Part model, mm, in its own coordinate system. A direction names the side the tool comes from. Give positions to 0.01 mm unless a question says otherwise; leave off trailing zeros. Write each loop counter-clockwise with the first axis right and the second up, starting at its lowest first coordinate (ties: lowest second). Pieces come first, ordered by that corner, then holes. Notation, with made-up numbers: M 82,75.25 L 111,75.25 A19 ccw 111,98.25 Z; hole C 35.5,22.5 d6. An arc over 180 degrees is marked long. Use CSV: the item, a comma, the result in double quotes. Start each with the question number.
Item 1: Cut at D-D (x = -14). List the corners of the cut face in (y, z), then the cut area to 3 significant figures.
Item 2: Cut at C-C (z = -1). List the corners of the cut face in (x, y).
Item 3: Mould opens along X. For faces 4 (the flat face through (19.646, 13.282, 3.535)), 5 (the flat face through (13.328, 19.691, 3.535)), 6 (the flat face through (19, -19, 1)), 7 (the cylindrical face through (-0.59, 4.46, -5.49)) say: released by +X, released by -X, zero draft, split by the parting line, or undercut.
Item 4: Pin check, flat tips, straight feed: pin 1 (18 mm diameter, centred on x = -3, y = -3, fed in from +Z); pin 2 (11 mm diameter, centred on x = 16.5, y = -19, fed in from -Z); pin 3 (1.5 mm diameter, centred on y = 16, z = 2.5, fed in from +X); pin 4 (3 mm diameter, centred on x = 17.75, y = 17.75, fed in from -Z). Stop position of each tip, or through.
Item 5: Drill centre lines: line 1 (X direction, y = -19.5, z = 2.5); line 2 (Y direction, x = 0, z = -1.4); line 3 (Z direction, x = -12.5, y = 2). Where is each one in solid material? Low to high. Write a range as [from, to].
Item 6: Which spindle directions (+Z, -Z, +X, -X, +Y, -Y) get a long thin tool onto all of the face, cutting with end or side? Do faces 1 (the cylindrical face through (-2.343, 17.847, 3.535)), 2 (the conical face through (21.2, -0.2, 5.8)), 3 (the flat face through (-19.5, 18.4, 1)). Say none if no direction does.
Item 7: Cut at A-A (y = 0). List the corners of the cut face in (x, z), then the cut area to 3 significant figures.
from build123d import *

# Parameters (mm, degrees)
SKETCH1_R           = 22
BOSS_EXTRUDE1_DEPTH = 6
CHAMFER1_SIZE       = 1
SKETCH8_R           = 1.6
BOSS_EXTRUDE2_DEPTH = 5
SKETCH9_R           = 18
CUT_EXTRUDE1_DEPTH  = 5
SKETCH10_R          = 8.5
CUT_EXTRUDE2_DEPTH  = 6
SKETCH11_R          = 4.5
CUT_EXTRUDE3_DEPTH  = 1


with BuildPart() as part:
    # Sketch1 → Boss-Extrude1 (new, symmetric)
    with BuildSketch(Plane.XY):
        Circle(SKETCH1_R)
    extrude(amount=BOSS_EXTRUDE1_DEPTH, both=True)

    # Chamfer1
    chamfer1_edges = [part.edges().sort_by_distance(p)[0] for p in [
        (-22, 0, 6),
    ]]
    chamfer(chamfer1_edges, length=CHAMFER1_SIZE)

    # Sketch8 → Boss-Extrude2 (add)
    # profile 1 of 4: a face of its own
    with BuildSketch(Plane.XY.offset(6)):
        with BuildLine():
            Line((20.930360723, -14.566399692), (17.68629022, -11.322329189))
            Line((17.68629022, -11.322329189), (11.322329189, -17.68629022))
            Line((11.322329189, -17.68629022), (14.566399692, -20.930360723))
            ThreePointArc((14.566399692, -20.930360723), (20.930360723, -20.930360723), (20.930360723, -14.566399692))
        make_face()
        with Locations((17.748380208, -17.748380208)):
            Circle(SKETCH8_R, mode=Mode.SUBTRACT)
    # profile 2 of 4: a face of its own
    with BuildSketch(Plane.XY.offset(6)):
        with BuildLine():
            Line((14.566399692, 20.930360723), (11.322329189, 17.68629022))
            Line((11.322329189, 17.68629022), (17.68629022, 11.322329189))
            Line((17.68629022, 11.322329189), (20.930360723, 14.566399692))
            ThreePointArc((20.930360723, 14.566399692), (20.930360723, 20.930360723), (14.566399692, 20.930360723))
        make_face()
        with Locations((17.748380208, 17.748380208)):
            Circle(SKETCH8_R, mode=Mode.SUBTRACT)
    # profile 3 of 4: a face of its own
    with BuildSketch(Plane.XY.offset(6)):
        with BuildLine():
            Line((-14.566399692, -20.930360723), (-11.322329189, -17.68629022))
            Line((-11.322329189, -17.68629022), (-17.68629022, -11.322329189))
            Line((-17.68629022, -11.322329189), (-20.930360723, -14.566399692))
            ThreePointArc((-20.930360723, -14.566399692), (-20.930360723, -20.930360723), (-14.566399692, -20.930360723))
        make_face()
        with Locations((-17.748380208, -17.748380208)):
            Circle(SKETCH8_R, mode=Mode.SUBTRACT)
    # profile 4 of 4: a face of its own
    with BuildSketch(Plane.XY.offset(6)):
        with BuildLine():
            Line((-20.930360723, 14.566399692), (-17.68629022, 11.322329189))
            Line((-17.68629022, 11.322329189), (-11.322329189, 17.68629022))
            Line((-11.322329189, 17.68629022), (-14.566399692, 20.930360723))
            ThreePointArc((-14.566399692, 20.930360723), (-20.930360723, 20.930360723), (-20.930360723, 14.566399692))
        make_face()
        with Locations((-17.748380208, 17.748380208)):
            Circle(SKETCH8_R, mode=Mode.SUBTRACT)
    extrude(amount=-BOSS_EXTRUDE2_DEPTH)

    # Sketch9 → Cut-Extrude1 (cut)
    with BuildSketch(Plane.XY.offset(6)):
        Circle(SKETCH9_R)
    extrude(amount=-CUT_EXTRUDE1_DEPTH, mode=Mode.SUBTRACT)

    # Sketch10 → Cut-Extrude2 (cut)
    with BuildSketch(Plane.XY.offset(1)):
        Circle(SKETCH10_R)
    extrude(amount=-CUT_EXTRUDE2_DEPTH, mode=Mode.SUBTRACT)

    # Sketch11 → Cut-Extrude3 (cut)
    with BuildSketch(Plane.XY.offset(-5)):
        Circle(SKETCH11_R)
    extrude(amount=-CUT_EXTRUDE3_DEPTH, mode=Mode.SUBTRACT)


solid = part.part
Worked answers:
1,outline,"M -20.36,1 L -16.97,1 L -16.97,-6 L 16.97,-6 L 16.97,1 L 20.36,1 L 20.36,6 L 11.31,6 L 11.31,1 L -11.31,1 L -11.31,6 L -20.36,6 Z"
1,area,"328 mm^2"
2,outline,"C 0,0 d44; hole C 0,0 d17"
3,face 4,"released by +X"
3,face 5,"undercut"
3,face 6,"zero draft"
3,face 7,"undercut"
4,pin 1,"stops at z = 1"
4,pin 2,"stops at z = -6"
4,pin 3,"stops at x = 22.14"
4,pin 4,"passes through"
5,line 1,"x = [-21.89, -13.14], [-10.19, 10.19], [13.14, 21.89]"
5,line 2,"y = [-22, -8.5], [8.5, 22]"
5,line 3,"z = [-6, 1]"
6,face 1,"+Z"
6,face 2,"+Z, +X"
6,face 3,"-Z, -X, +Y"
7,outline,"M -22,-6 L -4.5,-6 L -4.5,-5 L -8.5,-5 L -8.5,1 L -18,1 L -18,6 L -21,6 L -22,5 Z; M 4.5,-6 L 22,-6 L 22,5 L 21,6 L 18,6 L 18,1 L 8.5,1 L 8.5,-5 L 4.5,-5 Z"
7,area,"236 mm^2"
